from build123d import *

# Parameters (mm, degrees)
BOSS_EXTRUDE2_DEPTH = 72
SKETCH3_W           = 12
SKETCH3_H           = 40
CUT_EXTRUDE1_DEPTH  = 4
CUT_EXTRUDE2_DEPTH  = 116.296301893
SKETCH5_W           = 12
SKETCH5_H           = 13.444323502
CUT_EXTRUDE3_DEPTH  = 4
CHAMFER1_SIZE       = 3.2
FILLET1_R           = 3


with BuildPart() as part:
    # Sketch2 → Boss-Extrude2 (new body)
    with BuildSketch(Plane(origin=(0, 0, 0), x_dir=(0, 0, -1), z_dir=(1, 0, 0))):
        with BuildLine():
            Line((10.606601718, 40.606601718), (0, 30))
            Line((0, 30), (-42.426406871, 72.426406871))
            ThreePointArc((-42.426406871, 72.426406871), (-32.969757857, 33.917072276), (-53.513108843, 0))
            Line((-53.513108843, 0), (0, 0))
            Line((0, 0), (30, 0))
            Line((30, 0), (51.213203436, 0))
            Line((51.213203436, 0), (10.606601718, 40.606601718))
        make_face()
    extrude(amount=BOSS_EXTRUDE2_DEPTH)

    # Sketch3 → Cut-Extrude1 (cut)
    with BuildSketch(Plane(origin=(0, 25.606601718, -25.606601718), x_dir=(1, 0, 0), z_dir=(0, 0.7071067811865561, -0.7071067811865389))):
        with Locations((18, -1.213203436)):
            Rectangle(SKETCH3_W, SKETCH3_H)
    extrude(amount=-CUT_EXTRUDE1_DEPTH, mode=Mode.SUBTRACT)

    # Sketch4 → Cut-Extrude2 (cut, through all)
    with BuildSketch(Plane(origin=(72, 0, 0), x_dir=(0, 0, -1), z_dir=(1, 0, 0))):
        Polygon((0, 30), (17.67766953, 12.32233047), (28.284271247, 22.928932188), (10.606601718, 40.606601718), align=None)
    extrude(amount=-CUT_EXTRUDE2_DEPTH, mode=Mode.SUBTRACT)

    # Sketch5 → Cut-Extrude3 (cut)
    with BuildSketch(Plane(origin=(0, 25.606601718, -25.606601718), x_dir=(1, 0, 0), z_dir=(0, 0.7071067811865561, -0.7071067811865389))):
        with Locations((18, 25.508958315)):
            Rectangle(SKETCH5_W, SKETCH5_H)
    extrude(amount=-CUT_EXTRUDE3_DEPTH, mode=Mode.SUBTRACT)

    # Chamfer1
    chamfer1_edges = [part.edges().sort_by_distance(p)[0] for p in [
        (18, 2.815758154, -48.397445281),
    ]]
    chamfer(chamfer1_edges, length=CHAMFER1_SIZE)

    # Fillet1
    fillet1_edges = [part.edges().sort_by_distance(p)[0] for p in [
        (24, 10.050252532, -35.506096654),
        (12, 10.050252532, -35.506096654),
    ]]
    fillet(fillet1_edges, radius=FILLET1_R)


solid = part.part
Input: part model. Units: mm. Frame: model coordinates. A direction names the side the tool comes from. Coordinates: 2 decimals unless noted, no trailing zeros. Order: outer loops, then holes, each group sorted by start corner. A loop starts at its lowest first (then second) coordinate and runs counter-clockwise, first axis right, second up. Notation, with made-up numbers: M 55,-17.75 L 78,-17.75 A29 cw 78,18.25 Z; hole C 17,57 d8. An arc over 180 degrees is marked long. Answer in a Markdown table with one row per item.
(1) Material intervals for line 1 (Z direction, x = 46.5, y = 14); line 2 (Y direction, x = 20.5, z = -45); line 3 (Z direction, x = 7, y = 10), sorted ascending. Write a range as [from, to].
Numbers:
| item | result |
|---|---|
| line 1 | z = [-37.21, -19.36], [-16, 40.44] |
| line 2 | y = [0, 0.56] |
| line 3 | z = [-41.21, 43.25] |
(2) Section query A-A, the plane x = 18. Output: boundary loops of the cut face in (y, z), plus the area to 3 significant figures.
Numbers:
| item | result |
|---|---|
| outline | M 0,-51.21 L 0.55,-50.66 L 0.55,-46.13 L 0,-45.58 Z; M 0,-45.56 L 20.1,-25.46 L 12.32,-17.68 L 72.43,42.43 A51.81 cw 0,53.51 Z |
| area | 2,510 mm^2 |
(3) Contact query for flat-ended pins moving along their axis: pin 1 Ø12 at (y, z) = (38.5, -2.5) entering from -X; pin 2 Ø12 at (x, z) = (17, -18.5) entering from +Y; pin 3 Ø11 at (y, z) = (9, -44) entering from -X; pin 4 Ø12 at (x, z) = (30, 10) entering from +Y. Output: stop coordinate, or through.
Numbers:
| item | result |
|---|---|
| pin 1 | passes through |
| pin 2 | stops at y = 19.14 |
| pin 3 | stops at x = 0 |
| pin 4 | stops at y = 46 |
(4) Draft query along X for faces 4 (the flat face through (35.496, 11.304, -39.909)), 5 (the flat face through (72, 18, 9)), 6 (the flat face through (17.958, 9.91, -35.647)). Return one class per face: pulls with the +X half, pulls with the -X half, needs draft (parallel to the pull), parting line crosses it, or undercut.
Numbers:
| item | result |
|---|---|
| face 4 | needs draft |
| face 5 | pulls with the +X half |
| face 6 | undercut |
(5) Section query D-D, the plane y = 49. Output: boundary loops of the cut face in (x, z).
Numbers:
| item | result |
|---|---|
| outline | M 0,19 L 72,19 L 72,32.88 L 0,32.88 Z |
(6) Access query for faces 1 (the flat face through (18, 0.553, -48)), 2 (the flat face through (0, 18, 9)), 3 (the flat face through (35, 42, 12)). Directions: +Z, -Z, +X, -X, +Y, -Y. A direction counts if a zero-diameter tool reaches every point of the face in a straight line with its end or side. Return the directions, or none.
Numbers:
| item | result |
|---|---|
| face 1 | -Z, +Y |
| face 2 | +Z, -Z, -X, +Y, -Y |
| face 3 | +X, -X, +Y |
(7) Section query C-C, the plane x = 56. Output: boundary loops of the cut face in (y, z).
Numbers:
| item | result |
|---|---|
| outline | M 0,-51.21 L 22.93,-28.28 L 12.32,-17.68 L 72.43,42.43 A51.81 cw 0,53.51 Z |
(8) Section query B-B, the plane z = 13. Output: boundary loops of the cut face in (x, y), plus the area to 3 significant figures.
Numbers:
| item | result |
|---|---|
| outline | M 0,0 L 72,0 L 72,43 L 0,43 Z |
| area | 3,100 mm^2 |
